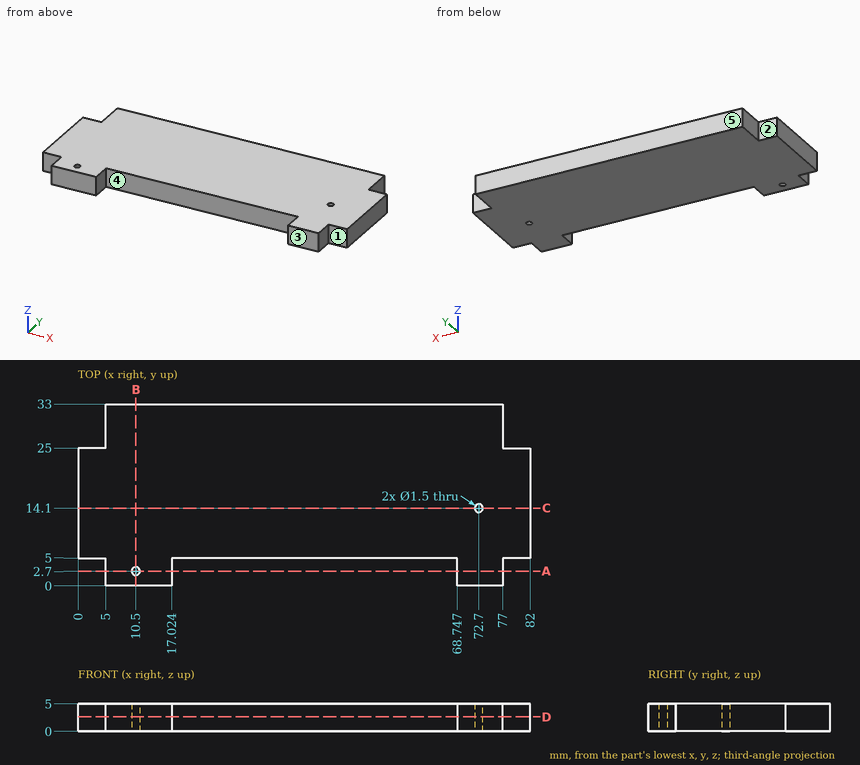
Verification items for this drawing (mm, ordinates from the low corner). A direction names the side the tool comes from. Coordinates: 2 decimals unless noted, no trailing zeros. Order: outer loops, then holes, each group sorted by start corner. A loop starts at its lowest first (then second) coordinate and runs counter-clockwise, first axis right, second up. Notation, with made-up numbers: M -1,32 L 34,32 A31 ccw 34,59 Z; hole C 76.25,-33 d11. An arc over 180 degrees is marked long. One line per item, written item: value. Start each with the question number.
Item 1: Sectioned sample at D-D on z = 2.65. Record the cut outline in (x, y).
Item 2: Depth check by flat-ended pin: P1, Ø1, axis at y = 29.5, z = 2, coming from the +X side; P2, Ø1.5, axis at x = 28.5, y = 7, coming from the -Z side; P3, Ø2.5, axis at x = 40.5, z = 2, coming from the -Y side; P4, Ø2.5, axis at y = 28, z = 2.5, coming from the -X side. Enter the tip coordinate at first touch or a pass-through.
Item 3: Mould release check, pull along X, two halves, no side actions. Record for the marked faces 4 and 5: pulls with the +X half, pulls with the -X half, needs draft (parallel to the pull), parting line crosses it, or undercut.
Item 4: Sectioned sample at C-C on y = 14.1. Record the cut outline in (x, z).
Item 5: Access from +Z, -Z, +X, -X, +Y, -Y to the whole of each face (thin tool, end or side, straight path). Record for the marked faces 1, 2 and 3.
Item 6: Sectioned sample at B-B on x = 10.5. Record the cut outline in (y, z).
Item 7: Sectioned sample at A-A on y = 2.7. Record the cut outline in (x, z).
Item 8: Thickness scan on probe 1 along Y at (x, z) = (10.5, 2.1); probe 2 along X at (y, z) = (2.5, 1.95); probe 3 along Y at (x, z) = (39, 3.75). Record the ranges inside material, lowest first.
Calculated:
1. outline: M 0,5 L 5,5 L 5,0 L 17.02,0 L 17.02,5 L 68.75,5 L 68.75,0 L 77,0 L 77,5 L 82,5 L 82,25 L 77,25 L 77,33 L 5,33 L 5,25 L 0,25 Z; hole C 10.5,2.7 d1.5; hole C 72.7,14.1 d1.5
2. P1: x = 77
2. P2: z = 0
2. P3: y = 5
2. P4: x = 5
3. face 4: undercut
3. face 5: needs draft
4. outline: M 0,0 L 71.95,0 L 71.95,5 L 0,5 Z; M 73.45,0 L 82,0 L 82,5 L 73.45,5 Z
5. face 1: +Z, -Z, +X, -Y
5. face 2: +Z, -Z, -X, +Y
5. face 3: +Z, -Z, +X, -X, -Y
6. outline: M 0,0 L 1.95,0 L 1.95,5 L 0,5 Z; M 3.45,0 L 33,0 L 33,5 L 3.45,5 Z
7. outline: M 5,0 L 9.75,0 L 9.75,5 L 5,5 Z; M 11.25,0 L 17.02,0 L 17.02,5 L 11.25,5 Z; M 68.75,0 L 77,0 L 77,5 L 68.75,5 Z
8. probe 1: 0 to 1.95, 3.45 to 33
8. probe 2: 5 to 9.78, 11.22 to 17.02, 68.75 to 77
8. probe 3: 5 to 33
